from build123d import *

# Parameters (mm, degrees)
SKETCH1_W           = 45.5
SKETCH1_H           = 20.5
BOSS_EXTRUDE1_DEPTH = 3
SKETCH2_R           = 8
BOSS_EXTRUDE2_DEPTH = 12
SKETCH3_W           = 10
SKETCH3_H           = 3
BOSS_EXTRUDE3_DEPTH = 11
SKETCH4_R           = 6.5
CUT_EXTRUDE1_DEPTH  = 1
FILLET1_R           = 15
SKETCH5_W           = 10
SKETCH5_H           = 3.5
BOSS_EXTRUDE4_DEPTH = 3
FILLET2_R           = 2


with BuildPart() as part:
    # Sketch1 → Boss-Extrude1 (new body)
    with BuildSketch(Plane(origin=(0, 0, 0), x_dir=(1, 0, 0), z_dir=(0, 1, 0))):
        with Locations((22.75, 10.25)):
            Rectangle(SKETCH1_W, SKETCH1_H)
    extrude(amount=BOSS_EXTRUDE1_DEPTH)

    # Sketch2 → Boss-Extrude2 (add)
    with BuildSketch(Plane(origin=(0, 3, 0), x_dir=(1, 0, 0), z_dir=(0, 1, 0))):
        with Locations(Location((10, 10.25, 0), (0, 0, 90))):
            Circle(SKETCH2_R)
        with Locations(Location((35.5, 10.25, 0), (0, 0, 90))):
            Circle(SKETCH2_R)
    extrude(amount=BOSS_EXTRUDE2_DEPTH)

    # Sketch3 → Boss-Extrude3 (add)
    with BuildSketch(Plane.XZ):
        with Locations((22.75, -2.5)):
            Rectangle(SKETCH3_W, SKETCH3_H)
    extrude(amount=BOSS_EXTRUDE3_DEPTH)

    # Sketch4 → Cut-Extrude1 (cut)
    with BuildSketch(Plane(origin=(0, 15, 0), x_dir=(1, 0, 0), z_dir=(0, 1, 0))):
        with Locations(Location((10, 10.25, 0), (0, 0, 270))):
            Circle(SKETCH4_R)
        with Locations(Location((35.5, 10.25, 0), (0, 0, 270))):
            Circle(SKETCH4_R)
    extrude(amount=-CUT_EXTRUDE1_DEPTH, mode=Mode.SUBTRACT)

    # Fillet1
    # the kernel refuses this fillet: 15 mm, written as the material it adds along each edge
    with BuildSketch(Plane(origin=(10, 14, -10.25), x_dir=(0, 0, 1), z_dir=(-1, 0, 0))) as fillet1_piece_1:
        with BuildLine():
            CenterArc((1.114835193, 15), FILLET1_R, 270, 21.039469781)
            Line((1.114835193, 0), (1.114835193, -0.3))
            Line((1.114835193, -0.3), (6.5, -0.3))
            Line((6.5, -0.3), (6.8, 0))
            ThreePointArc((6.8, 0), (6.8, 0.5), (6.607703296, 0.72))
            Line((6.607703296, 0.72), (6.5, 1))
        make_face()
    revolve(axis=Axis((10, 14, -10.25), (0, 1, 0)))
    with BuildSketch(Plane(origin=(35.5, 14, -10.25), x_dir=(0, 0, 1), z_dir=(-1, 0, 0))) as fillet1_piece_2:
        with BuildLine():
            CenterArc((1.114835193, 15), FILLET1_R, 270, 21.039469781)
            Line((1.114835193, 0), (1.114835193, -0.3))
            Line((1.114835193, -0.3), (6.5, -0.3))
            Line((6.5, -0.3), (6.8, 0))
            ThreePointArc((6.8, 0), (6.8, 0.5), (6.607703296, 0.72))
            Line((6.607703296, 0.72), (6.5, 1))
        make_face()
    revolve(axis=Axis((35.5, 14, -10.25), (0, 1, 0)))

    # Sketch5 → Boss-Extrude4 (add)
    with BuildSketch(Plane(origin=(0, 3, 0), x_dir=(1, 0, 0), z_dir=(0, 1, 0))):
        with Locations((22.75, 2.75)):
            Rectangle(SKETCH5_W, SKETCH5_H)
    extrude(amount=BOSS_EXTRUDE4_DEPTH)

    # Fillet2
    # the kernel refuses this fillet: 2 mm, written as the material it takes off along each edge
    with BuildSketch(Plane(origin=(17.75, 3, -1), x_dir=(0, 0, -1), z_dir=(0, 1, 0)), Plane(origin=(27.75, 3, -1), x_dir=(-1, 0, 0), z_dir=(0, 1, 0)), Plane(origin=(27.75, 3, -4.5), x_dir=(0, 0, 1), z_dir=(0, 1, 0))) as fillet2_piece_1:
        with BuildLine():
            CenterArc((FILLET2_R, -FILLET2_R), FILLET2_R, 90, 90)
            Line((0, -FILLET2_R), (0, 0))
            Line((0, 0), (FILLET2_R, 0))
        make_face()
    extrude(amount=8, mode=Mode.SUBTRACT)
    with BuildSketch(Plane(origin=(17.75, 3, -4.5), x_dir=(0, 0, 1), z_dir=(0, 1, 0))) as fillet2_piece_2:
        with BuildLine():
            CenterArc((FILLET2_R, FILLET2_R), FILLET2_R, 180, 90)
            Line((0, FILLET2_R), (0, 0))
            Line((0, 0), (FILLET2_R, 0))
        make_face()
    extrude(amount=8, mode=Mode.SUBTRACT)


solid = part.part
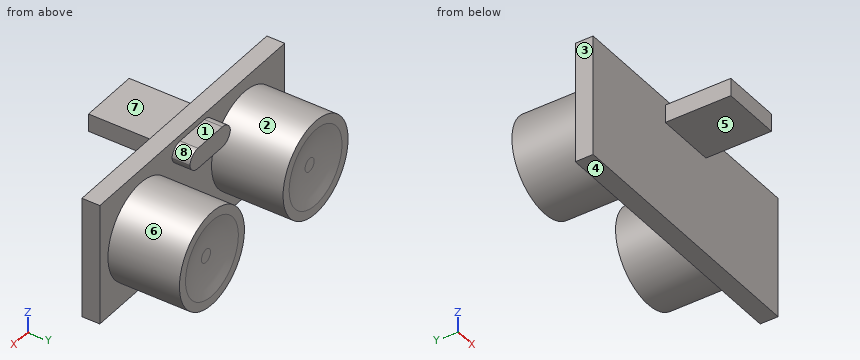
Work out the finished part from the listing and answer in its coordinate system (mm). Face numbers are marked on the shaded views. A direction names the side the tool comes from. Coordinates: 2 decimals unless noted, no trailing zeros. Write each loop counter-clockwise with the first axis right and the second up, starting at its lowest first coordinate (ties: lowest second). Pieces come first, ordered by that corner, then holes. Notation, with made-up numbers: M -35,66 L -17,66 A19 cw -17,97 Z; hole C 79,1 d3. An arc over 180 degrees is marked long. Use one line per item in the form item = value. Start each with the question number.
1. The part is cut by section A-A (y = 9.75). Give the vertices of the cut face in (x, z), plus the area to 3 significant figures.
2. Each of these flat-tipped pins is pushed along its axis until it touches: P1, Ø0.9, axis at x = 24, y = 4.5, coming from the +Z side; P2, Ø6, axis at x = 21.5, z = -8, coming from the -Y side; P3, Ø0.7, axis at x = 35.5, z = -10, coming from the +Y side; P4, Ø10, axis at x = 9.5, y = -7.5, coming from the +Z side. Where does it stop, or does it pass through?
3. Straight lines are drawn through the part: probe 1 along X at (y, z) = (3.75, -10.5); probe 2 along Y at (x, z) = (18.5, -0.75); probe 3 along Z at (x, y) = (21, -6). For each, find the intervals that lie inside material, in ascending order. Write a range as from..to.
4. A tool of negligible diameter and unlimited length cuts with its end or side. For the marked faces 4, 5, 6, 7 and 8, from which of +Z, -Z, +X, -X, +Y, -Y can it reach the whole face along a straight path? Write none if from no direction.
5. The mould has two halves that part along X. Classify the marked faces 1, 2 and 3: released by +X, released by -X, zero draft, split by the parting line, or undercut.
6. The part is cut by section B-B (y = -8). Give the vertices of the cut face in (x, z), plus the area to 3 significant figures.
Evaluation:
q1.outline = C 10,-10.25 d16; C 35.5,-10.25 d16
q1.area = 402 mm^2
q2.P1 = -1
q2.P2 = 0
q2.P3 = 14
q2.P4 = through
q3.probe_1 = 2..18, 27.5..43.5
q3.probe_2 = 0..3
q3.probe_3 = -4..-1
q4.face_4 = -Z, +X, -X, +Y, -Y
q4.face_5 = -Z, +X, -X, -Y
q4.face_6 = +Y
q4.face_7 = +Z, +X, -X, -Y
q4.face_8 = +Z, +Y
q5.face_1 = zero draft
q5.face_2 = undercut
q5.face_3 = released by -X
q6.outline = M 17.75,-4 L 27.75,-4 L 27.75,-1 L 17.75,-1 Z
q6.area = 30.0 mm^2
